from build123d import *

# Parameters (mm, degrees)
SKETCH2_W           = 78
SKETCH2_H           = 63
BOSS_EXTRUDE1_DEPTH = 10
SKETCH3_W           = 74.327682065
SKETCH3_H           = 59
CUT_EXTRUDE1_DEPTH  = 8
CUT_EXTRUDE2_DEPTH  = 0.5
SKETCH7_R           = 1
CUT_EXTRUDE4_DEPTH  = 10


with BuildPart() as part:
    # Sketch2 → Boss-Extrude1 (new body)
    with BuildSketch(Plane(origin=(0, 0, 0), x_dir=(1, 0, 0), z_dir=(0, 1, 0))):
        with Locations((2.333333333, -2.169871795)):
            Rectangle(SKETCH2_W, SKETCH2_H)
    extrude(amount=BOSS_EXTRUDE1_DEPTH)

    # Sketch3 → Cut-Extrude1 (cut)
    with BuildSketch(Plane(origin=(0, 10, 0), x_dir=(1, 0, 0), z_dir=(0, 1, 0))):
        with Locations((2.497174366, -2.169871795)):
            Rectangle(SKETCH3_W, SKETCH3_H)
    extrude(amount=-CUT_EXTRUDE1_DEPTH, mode=Mode.SUBTRACT)

    # Sketch6 → Cut-Extrude2 (cut)
    with BuildSketch(Plane.XZ):
        with BuildLine():
            Line((32.690802989, -22.584376441), (33.092200105, -22.584376441))
            ThreePointArc((33.092200105, -22.584376441), (33.114100993, -22.618218468), (33.137410711, -22.651105984))
            Line((33.137410711, -22.651105984), (32.08626128, -24.407558571))
            Line((32.08626128, -24.407558571), (29.226689091, -24.966180766))
            Line((29.226689091, -24.966180766), (30.376407219, -24.966180766))
            Line((30.376407219, -24.966180766), (32.232099133, -24.678141196))
            Line((32.232099133, -24.678141196), (33.226175577, -23.014639973))
            Line((33.226175577, -23.014639973), (33.137410711, -24.966180766))
            Line((33.137410711, -24.966180766), (30.816462944, -26.648982972))
            Line((30.816462944, -26.648982972), (32.08626128, -26.016434732))
            Line((32.08626128, -26.016434732), (33.372391781, -25.083926351))
            Line((33.372391781, -25.083926351), (33.526915315, -22.957480273))
            Line((33.526915315, -22.957480273), (34.264738027, -25.146278223))
            Line((34.264738027, -25.146278223), (36.880788863, -26.733349716))
            Line((36.880788863, -26.733349716), (36.19146957, -26.016434732))
            Line((36.19146957, -26.016434732), (34.598609497, -24.966180766))
            Line((34.598609497, -24.966180766), (33.944592444, -23.148589195))
            Line((33.944592444, -23.148589195), (35.243832983, -24.678141196))
            Line((35.243832983, -24.678141196), (38.980139277, -25.248190523))
            Line((38.980139277, -25.248190523), (37.817752325, -24.735025947))
            Line((37.817752325, -24.735025947), (35.578982945, -24.393456258))
            Line((35.578982945, -24.393456258), (34.251613969, -22.972216889))
            Line((34.251613969, -22.972216889), (34.631588177, -22.701732047))
            ThreePointArc((34.631588177, -22.701732047), (38.008201605, -22.081175269), (34.631149946, -21.463007775))
            Line((34.631149946, -21.463007775), (34.32916984, -21.227330494))
            Line((34.32916984, -21.227330494), (35.531005717, -19.871495744))
            Line((35.531005717, -19.871495744), (37.865688927, -19.500837177))
            Line((37.865688927, -19.500837177), (39.115173896, -18.968080087))
            Line((39.115173896, -18.968080087), (35.279154236, -19.577093569))
            Line((35.279154236, -19.577093569), (33.904618441, -21.127757375))
            Line((33.904618441, -21.127757375), (34.598609497, -19.132922738))
            Line((34.598609497, -19.132922738), (36.19146957, -18.215735483))
            Line((36.19146957, -18.215735483), (36.894373516, -17.458564394))
            Line((36.894373516, -17.458564394), (34.287546919, -18.959605302))
            Line((34.287546919, -18.959605302), (33.521005252, -21.208203232))
            Line((33.521005252, -21.208203232), (33.521005252, -19.132922738))
            Line((33.521005252, -19.132922738), (32.128586258, -17.983657476))
            Line((32.128586258, -17.983657476), (30.914042032, -17.358519989))
            Line((30.914042032, -17.358519989), (33.20673173, -19.250844523))
            Line((33.20673173, -19.250844523), (33.250345457, -21.088483091))
            Line((33.250345457, -21.088483091), (32.358416357, -19.616940759))
            Line((32.358416357, -19.616940759), (30.157760841, -19.132922738))
            Line((30.157760841, -19.132922738), (29.226689091, -19.196288455))
            Line((29.226689091, -19.196288455), (32.08626128, -19.82523036))
            Line((32.08626128, -19.82523036), (33.137410711, -21.514148052))
            ThreePointArc((33.137410711, -21.514148052), (33.108673975, -21.555134418), (33.0821246, -21.597570405))
            Line((33.0821246, -21.597570405), (32.690802989, -21.597570405))
            Line((32.690802989, -21.597570405), (32.334590078, -21.674589412))
            Line((32.334590078, -21.674589412), (32.334590078, -21.93528367))
            Line((32.334590078, -21.93528367), (32.490652027, -21.862323244))
            Line((32.490652027, -21.862323244), (32.961131868, -21.935626601))
            ThreePointArc((32.961131868, -21.935626601), (32.949905472, -22.099923891), (32.967075812, -22.263706708))
            Line((32.967075812, -22.263706708), (32.490652027, -22.355724574))
            Line((32.490652027, -22.355724574), (32.320109644, -22.245819483))
            Line((32.320109644, -22.245819483), (32.334590078, -22.512171121))
            Line((32.334590078, -22.512171121), (32.690802989, -22.584376441))
        make_face()
    extrude(amount=-CUT_EXTRUDE2_DEPTH, mode=Mode.SUBTRACT)

    # Sketch7 → Cut-Extrude4 (cut)
    with BuildSketch(Plane.XZ):
        with Locations((-29.946640044, 2.169871795)):
            Circle(SKETCH7_R)
    extrude(amount=-CUT_EXTRUDE4_DEPTH, mode=Mode.SUBTRACT)


solid = part.part
Geometry: final body of the model. Coordinates: model frame, mm. A direction names the side the tool comes from. Coordinates: 2 decimals unless noted, no trailing zeros. Order: outer loops, then holes, each group sorted by start corner. A loop starts at its lowest first (then second) coordinate and runs counter-clockwise, first axis right, second up. Notation, with made-up numbers: (-31.5, 55) - (20.5, 55) arc R3 cw to (20.5, 59) - close; hole circle Ø3 at (30.25, -15.5). An arc over 180 degrees is marked (long way). Use one line per item in the form item = value.
1) Ray query, L1, parallel to X at y = 4.5, z = 26.5; L2, parallel to Z at x = 12, y = 8.5; L3, parallel to Y at x = 35.5, z = -10. Return the intervals inside material, ascending.
Solutions:
L1 = -36.67 to -34.67, 39.66 to 41.33
L2 = -29.33 to -27.33, 31.67 to 33.67
L3 = 0 to 2
2) Set-up query: faces 1 (the face through (41.333, 5, 3)), 2 (the face through (38.007, 0.246, -22.149)), 3 (the face through (2, 2, 2)). Return all of +Z, -Z, +X, -X, +Y, -Y with unobstructed straight access to the full face (end or side cutting, diameter ignored); none if empty.
Solutions:
face_1 = +Z, -Z, +X, +Y, -Y
face_2 = -Y
face_3 = +Y
3) Pin query (flat end, axial travel): pin 1 (1 mm diameter, centred on x = 7.5, z = 6, fed in from +Y); pin 2 (1.8 mm diameter, centred on x = -29.95, z = 2.17, fed in from +Y). Return the tip coordinate at first contact, or that it passes through.
Solutions:
pin_1 = 2
pin_2 = through
4) Section A-A (y = 5). Return loops of the section in (x, z), then the cut area to 3 significant figures.
Solutions:
outline = (-36.67, -29.33) - (41.33, -29.33) - (41.33, 33.67) - (-36.67, 33.67) - close; hole (-34.67, -27.33) - (39.66, -27.33) - (39.66, 31.67) - (-34.67, 31.67) - close
area = 529 mm^2
5) Section B-B (z = 26). Return loops of the section in (x, y), then the cut area to 3 significant figures.
Solutions:
outline = (-36.67, 0) - (41.33, 0) - (41.33, 10) - (39.66, 10) - (39.66, 2) - (-34.67, 2) - (-34.67, 10) - (-36.67, 10) - close
area = 185 mm^2
6) Section C-C (x = 15.5). Return loops of the section in (y, z).
Solutions:
outline = (0, -29.33) - (10, -29.33) - (10, -27.33) - (2, -27.33) - (2, 31.67) - (10, 31.67) - (10, 33.67) - (0, 33.67) - close
7) Mould query, pull axis X, two halves, no side actions, for faces 4 (the face through (2, 5, -29.33)), 5 (the face through (-36.667, 5, 3)), 6 (the face through (35.554, 0.246, -25.929)). Classes: +X half, -X half, draft (parallel to the pull), parting line (faces both ways), or undercut.
Solutions:
face_4 = draft
face_5 = -X half
face_6 = undercut
